Input: part model. Units: mm. Frame: model coordinates. Give positions to 0.01 mm unless a question says otherwise; leave off trailing zeros. Loops run counter-clockwise (first coordinate to the right, second up) from the corner with the lowest first, then second, coordinate; pieces in that order, holes last. Notation, with made-up numbers: M 19.25,-1.75 L 49.25,-1.75 A26 ccw 49.25,12.25 Z; hole C 70.25,-13 d5. An arc over 180 degrees is marked long. Use a Markdown table: item, result. Add a question column.
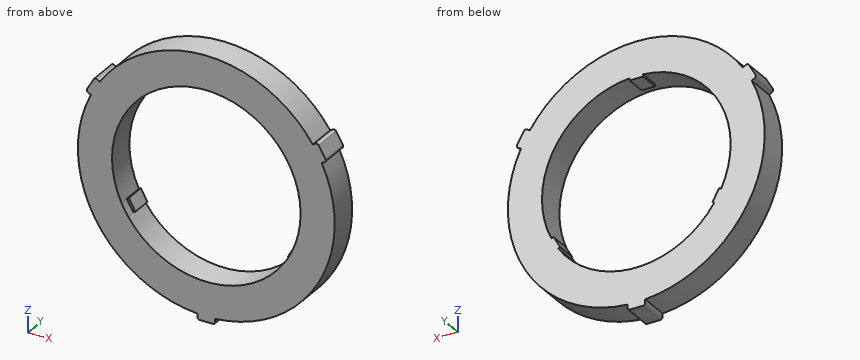
from build123d import *
from build123d.topology import SkipClean

# Parameters (mm, degrees)
BOSS_EXTRUDE1_DEPTH = 6.5
FILLET1_R           = 0.5
CUT_EXTRUDE1_DEPTH  = 2


with BuildPart() as part:
    # Sketch1 → Boss-Extrude1 (new body)
    with BuildSketch(Plane(origin=(0, 0, 0), x_dir=(1, 0, 0), z_dir=(0, 1, 0))):
        with BuildLine():
            ThreePointArc((25.881318293, -12.633185007), (24.941531629, 14.4), (2, 28.730471629))
            Line((2, 28.730471629), (2, 30))
            Line((2, 30), (-2, 30))
            Line((-2, 30), (-2, 28.730471629))
            ThreePointArc((-2, 28.730471629), (-24.941531629, 14.4), (-25.881318293, -12.633185007))
            Line((-25.881318293, -12.633185007), (-26.980762114, -13.267949192))
            Line((-26.980762114, -13.267949192), (-24.980762114, -16.732050808))
            Line((-24.980762114, -16.732050808), (-23.881318293, -16.097286622))
            ThreePointArc((-23.881318293, -16.097286622), (0, -28.8), (23.881318293, -16.097286622))
            Line((23.881318293, -16.097286622), (24.980762114, -16.732050808))
            Line((24.980762114, -16.732050808), (26.980762114, -13.267949192))
            Line((26.980762114, -13.267949192), (25.881318293, -12.633185007))
        make_face()
        with BuildLine():
            ThreePointArc((-1.5, -21.096741455), (-18.31643729, -10.575), (-19.020314037, 9.249332622))
            Line((-19.020314037, 9.249332622), (-18.590123318, 9.000961894))
            Line((-18.590123318, 9.000961894), (-17.090123318, 11.599038106))
            Line((-17.090123318, 11.599038106), (-17.520314037, 11.847408833))
            ThreePointArc((-17.520314037, 11.847408833), (0, 21.15), (17.520314037, 11.847408833))
            Line((17.520314037, 11.847408833), (17.090123318, 11.599038106))
            Line((17.090123318, 11.599038106), (18.590123318, 9.000961894))
            Line((18.590123318, 9.000961894), (19.020314037, 9.249332622))
            ThreePointArc((19.020314037, 9.249332622), (18.31643729, -10.575), (1.5, -21.096741455))
            Line((1.5, -21.096741455), (1.5, -20.6))
            Line((1.5, -20.6), (-1.5, -20.6))
            Line((-1.5, -20.6), (-1.5, -21.096741455))
        make_face(mode=Mode.SUBTRACT)
    extrude(amount=BOSS_EXTRUDE1_DEPTH)

    # Fillet1
    fillet1_edges = [part.edges().sort_by_distance(p)[0] for p in [
        (-24.980762114, 3.25, 16.732050808),
        (-26.980762114, 3.25, 13.267949192),
        (-2, 3.25, -30),
        (2, 3.25, -30),
        (26.980762114, 3.25, 13.267949192),
        (24.980762114, 3.25, 16.732050808),
    ]]
    fillet(fillet1_edges, radius=FILLET1_R)

    # Sketch1<5> → Cut-Extrude1 (cut)
    with SkipClean():  # the faces are left unmerged after this step: merging them gives an invalid solid
        with BuildSketch(Plane(origin=(0, 0, 0), x_dir=(1, 0, 0), z_dir=(0, 1, 0))):
            with BuildLine():
                Line((-1.5, -20.6), (-1.5, -21.096741455))
                ThreePointArc((-1.5, -21.096741455), (0, -21.15), (1.5, -21.096741455))
                Line((1.5, -21.096741455), (1.5, -20.6))
                Line((1.5, -20.6), (-1.5, -20.6))
            make_face()
            with BuildLine():
                ThreePointArc((-17.520314037, 11.847408833), (-18.31643729, 10.575), (-19.020314037, 9.249332622))
                Line((-19.020314037, 9.249332622), (-18.590123318, 9.000961894))
                Line((-18.590123318, 9.000961894), (-17.090123318, 11.599038106))
                Line((-17.090123318, 11.599038106), (-17.520314037, 11.847408833))
            make_face()
            with BuildLine():
                Line((18.590123318, 9.000961894), (19.020314037, 9.249332622))
                ThreePointArc((19.020314037, 9.249332622), (18.31643729, 10.575), (17.520314037, 11.847408833))
                Line((17.520314037, 11.847408833), (17.090123318, 11.599038106))
                Line((17.090123318, 11.599038106), (18.590123318, 9.000961894))
            make_face()
        extrude(amount=CUT_EXTRUDE1_DEPTH, mode=Mode.SUBTRACT)


solid = part.part
1) Contact query for flat-ended pins moving along their axis: P1, Ø0.6, axis at x = 17.5, z = -10.5, coming from the -Y side; P2, Ø0.5, axis at y = 5, z = 21, coming from the -X side. Output: stop coordinate, or through.
2) Section query B-B, the plane y = 1.25. Return the cut outline in (x, z).
3) Section query C-C, the plane z = -1. Return the cut outline in (x, y).
4) Ray query, line 1 (X direction, y = 1.5, z = 0); line 2 (Z direction, x = -8, y = 1.75); line 3 (Z direction, x = -13, y = 6.25). Return the intervals inside material, ascending. Write a range as [from, to].
5) Section query A-A, the plane x = 7.5. Return the cut outline in (y, z).
Entries:
| question | item | result |
|---|---|---|
| 1 | P1 | stops at y = 2 |
| 1 | P2 | stops at x = -19.97 |
| 2 | outline | M -26.73,13.7 A0.5 ccw -26.55,13.02 L -25.88,12.63 A28.8 ccw -2,-28.73 L -2,-29.5 A0.5 ccw -1.5,-30 L 1.5,-30 A0.5 ccw 2,-29.5 L 2,-28.73 A28.8 ccw 25.88,12.63 L 26.55,13.02 A0.5 ccw 26.73,13.7 L 25.23,16.3 A0.5 ccw 24.55,16.48 L 23.88,16.1 A28.8 ccw -23.88,16.1 L -24.55,16.48 A0.5 ccw -25.23,16.3 Z; hole C 0,0 d42.3 |
| 3 | outline | M -28.78,0 L -21.13,0 L -21.13,6.5 L -28.78,6.5 Z; M 21.13,0 L 28.78,0 L 28.78,6.5 L 21.13,6.5 Z |
| 4 | line 1 | x = [-28.8, -21.15], [21.15, 28.8] |
| 4 | line 2 | z = [-27.67, -19.58], [19.58, 27.67] |
| 4 | line 3 | z = [-25.7, -16.68], [16.68, 25.7] |
| 5 | outline | M 0,-27.81 L 6.5,-27.81 L 6.5,-19.78 L 0,-19.78 Z; M 0,19.78 L 6.5,19.78 L 6.5,27.81 L 0,27.81 Z |
